For this review, use the dimensioned drawing (mm, ordinates from the lowest corner) and the shaded views. A direction names the side the tool comes from. Coordinates: 2 decimals unless noted, no trailing zeros. Write each loop counter-clockwise with the first axis right and the second up, starting at its lowest first coordinate (ties: lowest second). Pieces come first, ordered by that corner, then holes.
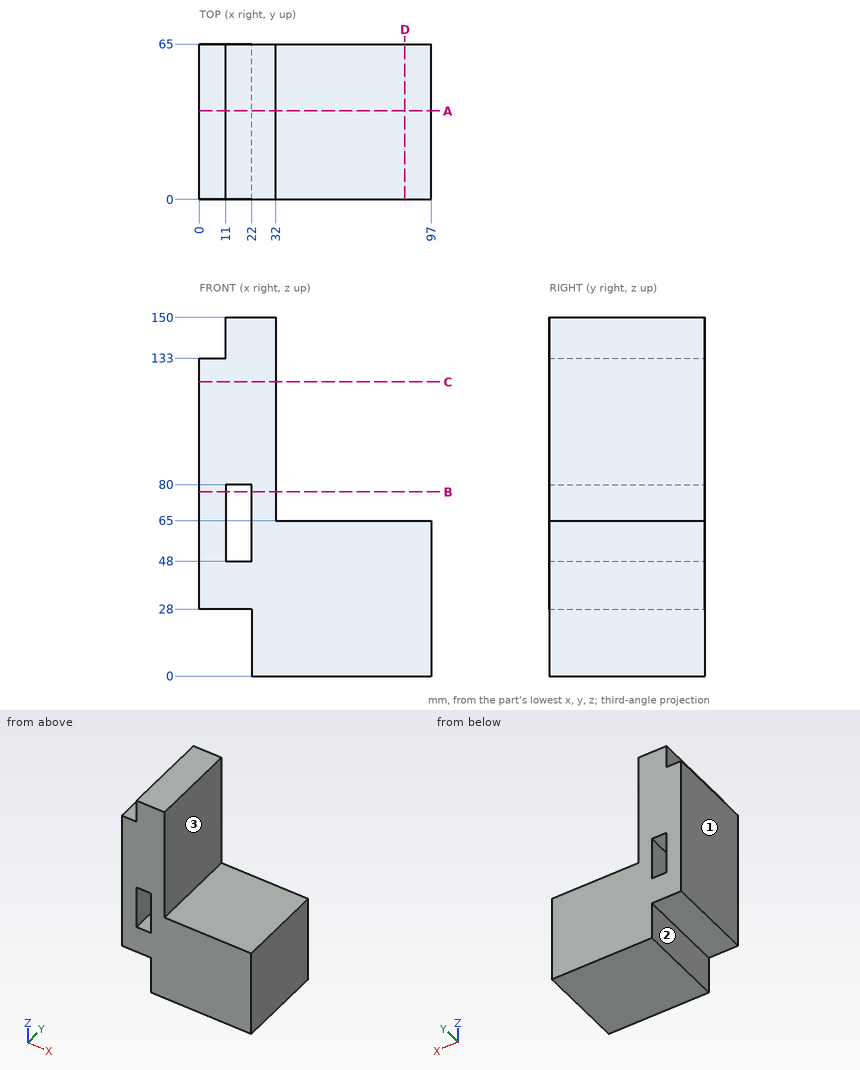
Item 1: To check wall thickness, follow line 1 along X through (y, z) = (55, 53); line 2 along X through (y, z) = (20, 79.5); line 3 along Z through (x, y) = (15, 46). State the ranges of each line that lie inside material, in increasing order.
Solved:
line 1: x = 0 to 11, 22 to 97
line 2: x = 0 to 11, 22 to 32
line 3: z = 28 to 48, 80 to 150
Item 2: Take a section at B-B, the plane z = 77. Write out the cut boundary in (x, y), plus the area to 4 significant figures.
Solved:
outline: (0, 0) - (11, 0) - (11, 65) - (0, 65) - close; (22, 0) - (32, 0) - (32, 65) - (22, 65) - close
area: 1,365 mm2
Item 3: Take a section at C-C, the plane z = 123. Write out the cut boundary in (x, y).
Solved:
outline: (0, 0) - (32, 0) - (32, 65) - (0, 65) - close
Item 4: For pin 1 (12 mm diameter, centred on x = 15.5, y = 25, fed in from -Z); pin 2 (8.5 mm diameter, centred on y = 39, z = 141, fed in from -X); pin 3 (4 mm diameter, centred on y = 28, z = 87, fed in from +X), all flat-tipped, find the tip position at first contact; note any pin that passes through.
Solved:
pin 1: stops at z = 28
pin 2: stops at x = 11
pin 3: stops at x = 32
Item 5: Take a section at A-A, the plane y = 37. Write out the cut boundary in (x, z), plus the area to 3 significant figures.
Solved:
outline: (0, 28) - (22, 28) - (22, 0) - (97, 0) - (97, 65) - (32, 65) - (32, 150) - (11, 150) - (11, 133) - (0, 133) - close; hole (11, 48) - (22, 48) - (22, 80) - (11, 80) - close
area: 7,870 mm2
Item 6: Machinability: for the marked faces 1, 2 and 3, which of the approach directions +Z, -Z, +X, -X, +Y, -Y give a long, thin tool a straight path to every point of the face, cutting with its end or side? Answer none if there is none.
Solved:
face 1: +Z, -Z, -X, +Y, -Y
face 2: -Z, -X, +Y, -Y
face 3: +Z, +X, +Y, -Y
Item 7: Take a section at D-D, the plane x = 86. Write out the cut boundary in (y, z).
Solved:
outline: (0, 0) - (65, 0) - (65, 65) - (0, 65) - close
